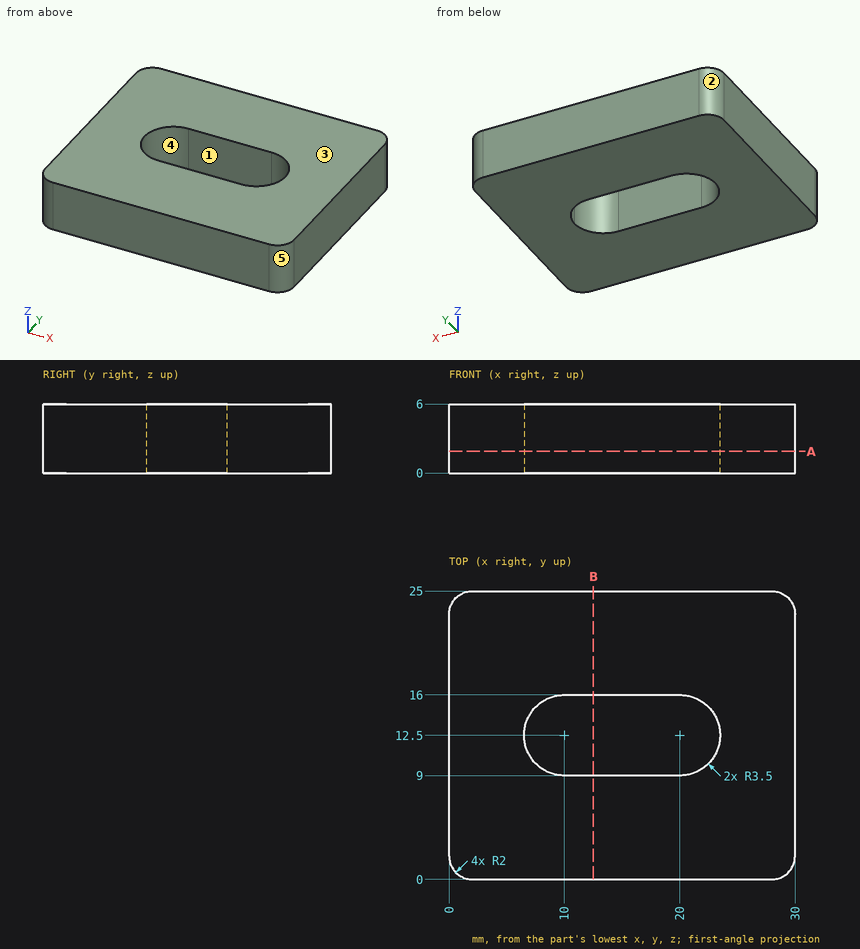
Geometry check sheet. Reference: drawing and pictorial views, mm from the part's lowest x, y, z. A direction names the side the tool comes from. Round coordinates to 2 decimals unless told otherwise and drop trailing zeros. Write each loop counter-clockwise with the first axis right and the second up, starting at its lowest first coordinate (ties: lowest second). Pieces come first, ordered by that corner, then holes.
Item 1: Access from +Z, -Z, +X, -X, +Y, -Y to the whole of each face (thin tool, end or side, straight path). Record for the marked faces 1 and 2.
Determined:
face 1: +Z, -Z
face 2: +Z, -Z, -X, +Y
Item 2: Go/stop test with a flat-tipped pin: pin 1 Ø6 at (x, y) = (16, 7.5) entering from -Z. Record where the tip stops, or that it passes through.
Determined:
pin 1: stops at z = 0
Item 3: Section check B-B (x = 12.5). Record the boundary of the cut face in (y, z), plus the area to 3 significant figures.
Determined:
outline: (0, 0) - (9, 0) - (9, 6) - (0, 6) - close; (16, 0) - (25, 0) - (25, 6) - (16, 6) - close
area: 108 mm2
Item 4: Mould release check, pull along X, two halves, no side actions. Record for the marked faces 3, 4 and 5: +X half, -X half, draft (parallel to the pull), parting line (faces both ways), or undercut.
Determined:
face 3: draft
face 4: undercut
face 5: +X half
Item 5: Material ranges on line 1 along Y through (x, z) = (18.5, 0.5); line 2 along Y through (x, z) = (22.5, 1.35); line 3 along X through (y, z) = (12.5, 1.6), recorded low to high.
Determined:
line 1: y = 0 to 9, 16 to 25
line 2: y = 0 to 10.05, 14.95 to 25
line 3: x = 0 to 6.5, 23.5 to 30
Item 6: Section check A-A (z = 1.9). Record the boundary of the cut face in (x, y), plus the area to 3 significant figures.
Determined:
outline: (0, 2) arc R2 ccw to (2, 0) - (28, 0) arc R2 ccw to (30, 2) - (30, 23) arc R2 ccw to (28, 25) - (2, 25) arc R2 ccw to (0, 23) - close; hole (10, 9) - (20, 9) arc R3.5 ccw to (20, 16) - (10, 16) arc R3.5 ccw to start
area: 638 mm2
